Verification items for the finished model (mm, model axes). A direction names the side the tool comes from. Coordinates: 2 decimals unless noted, no trailing zeros. Loops run counter-clockwise (first coordinate to the right, second up) from the corner with the lowest first, then second, coordinate; pieces in that order, holes last. Notation, with made-up numbers: (-34, -14.5) -> (13, -14.5) arc R31 ccw to (13, 12.5) -> close; hole circle Ø7 at (44.5, -31). An arc over 180 degrees is marked (long way). Write item = value, one per line.
```python
from build123d import *

# Parameters (mm, degrees)
BOX_W             = 7
BOX_H             = 7
BOX_DEPTH         = 7
ARRAY_COUNT       = 8
CYLINDER002_R     = 15
CYLINDER002_DEPTH = 10
CYLINDER001_R     = 20
CYLINDER001_DEPTH = 20
CYLINDER_R        = 20
CYLINDER_DEPTH    = 50


with BuildPart() as array:
    # Box → Box (new body)
    with BuildSketch(Plane(origin=(14, -3, 57), x_dir=(1, 0, 0), z_dir=(0, 0, 1))):
        with Locations((3.5, 3.5)):
            Rectangle(BOX_W, BOX_H)
    extrude(amount=BOX_DEPTH)

    # Array: Array ×8 about axis
    array_axis = Axis((0, 0, 0), (0, 0, 1))


with BuildPart() as array_1:
    add(array.part)
    for i in range(1, ARRAY_COUNT):
        add(array.part.rotate(array_axis, i * 360 / ARRAY_COUNT))


with BuildPart() as array_2:
    # Array placement: moved
    add(array_1.part.moved(Location((0, 0, -2))))


with BuildPart() as cilindre002:
    # Cylinder002 → Cylinder002 (new body)
    with BuildSketch(Plane.XY.offset(50)):
        Circle(CYLINDER002_R)
    extrude(amount=CYLINDER002_DEPTH)


with BuildPart() as cut:
    # Cylinder001 → Cylinder001 (new body)
    with BuildSketch(Plane.XY.offset(40)):
        Circle(CYLINDER001_R)
    extrude(amount=CYLINDER001_DEPTH)

    # Cut: cut Cilindre002
    add(cilindre002.part, mode=Mode.SUBTRACT)


with BuildPart() as cut001:
    # Cylinder → Cylinder (new body)
    with BuildSketch(Plane.XY):
        Circle(CYLINDER_R)
    extrude(amount=CYLINDER_DEPTH)

    # Fusion: union Cut
    add(cut.part)

    # Cut001: cut Array
    add(array_2.part, mode=Mode.SUBTRACT)


solid = cut001.part
```
1) Tool access check on faces 1 (the face through (-17, -4, 57)), 2 (the face through (13, -12, 55)), 3 (the face through (4, -17, 57)), 4 (the face through (14.28, 10.04, 57.46)). Record the directions out of +Z, -Z, +X, -X, +Y, -Y that give a thin tool (end or side, any length) a straight path to the whole face; none if there is none.
Ans:
face_1 = +Z, -X
face_2 = +Z
face_3 = +Z, -Y
face_4 = +Z, +Y
2) Sectioned sample at A-A, the plane y = 0. Record the cut outline in (x, z), plus the area to 3 significant figures.
Ans:
outline = (-20, 0) -> (20, 0) -> (20, 55) -> (15, 55) -> (15, 50) -> (-15, 50) -> (-15, 55) -> (-20, 55) -> close
area = 2,050 mm2
3) Sectioned sample at D-D, the plane y = -9.5. Record the cut outline in (x, z), plus the area to 3 significant figures.
Ans:
outline = (-17.6, 0) -> (17.6, 0) -> (17.6, 60) -> (15.16, 60) -> (15.16, 55) -> (11.61, 55) -> (11.61, 50) -> (-11.61, 50) -> (-11.61, 55) -> (-13.74, 55) -> (-13.74, 60) -> (-17.6, 60) -> close
area = 1,850 mm2
4) Depth check by flat-ended pin: pin 1 Ø1.5 at (y, z) = (17.5, 57.5) entering from +X; pin 2 Ø2.5 at (x, z) = (-16, 56.5) entering from -Y; pin 3 Ø4 at (y, z) = (8.5, 28.5) entering from +X. Enter the tip coordinate at first touch or a pass-through.
Ans:
pin_1 = 10.93
pin_2 = -11.86
pin_3 = 18.91
5) Sectioned sample at C-C, the plane z = 43.5. Record the cut outline in (x, y).
Ans:
outline = circle Ø40 at (0, 0)
6) Material ranges on line 1 (Y direction, x = 0, z = 52); line 2 (Z direction, x = 0.5, y = 14.5); line 3 (Y direction, x = 0.5, z = 21.5), recorded low to high.
Ans:
line_1 = -20 to -15, 15 to 20
line_2 = 0 to 50
line_3 = -19.99 to 19.99
7) Release check for a two-part mould opening along X. For faces 5 (the face through (-10.04, 14.28, 57.46)), 6 (the face through (14.842, -9.186, 57.465)), 7 (the face through (17, 1, 55)) record: pulls with the +X half, pulls with the -X half, needs draft (parallel to the pull), parting line crosses it, or undercut.
Ans:
face_5 = pulls with the -X half
face_6 = undercut
face_7 = needs draft
